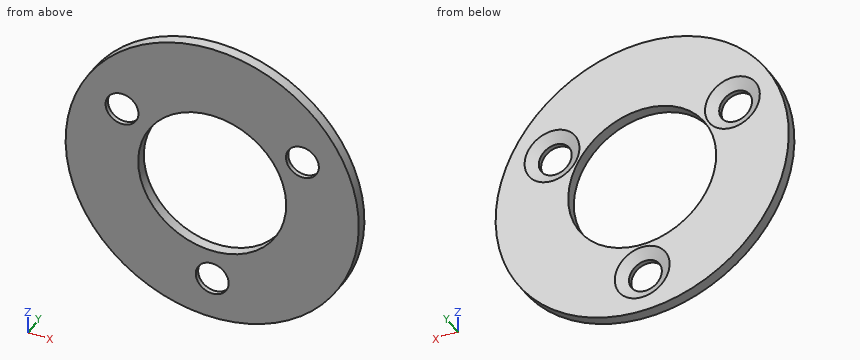
```python
from build123d import *

# Parameters (mm, degrees)
SKETCH_1_R          = 13.371753228
SKETCH_1_R_2        = 6.75
EXTRUDE_1_DEPTH     = 1
SKETCH_2_R          = 1.5
CUT_EXTRUDE_1_DEPTH = 2
CHAMFER_1_SIZE      = 1
CHAMFER_1_SIZE2     = 0.577350269


with BuildPart() as part:
    # 草图1 → 凸台-拉伸1 (new body)
    with BuildSketch(Plane(origin=(0, 0, 0), x_dir=(1, 0, 0), z_dir=(0, 1, 0))):
        with Locations(Location((0, 0, 0), (0, 0, 270))):
            Circle(SKETCH_1_R)
        with Locations(Location((0, 0, 0), (0, 0, 270))):
            Circle(SKETCH_1_R_2, mode=Mode.SUBTRACT)
    extrude(amount=EXTRUDE_1_DEPTH)

    # 草图2 → 切除-拉伸1 (cut)
    with BuildSketch(Plane(origin=(0, 1, 0), x_dir=(1, 0, 0), z_dir=(0, 1, 0))):
        with Locations(Location((0, 9.5, 0), (0, 0, 270))):
            Circle(SKETCH_2_R)
        with Locations(Location((8.227241336, -4.75, 0), (0, 0, 270))):
            Circle(SKETCH_2_R)
        with Locations(Location((-8.227241336, -4.75, 0), (0, 0, 270))):
            Circle(SKETCH_2_R)
    extrude(amount=-CUT_EXTRUDE_1_DEPTH, mode=Mode.SUBTRACT)

    # 倒角1
    chamfer_1_edges = [part.edges().sort_by_distance(p)[0] for p in [
        (0, 1, -11),
        (8.227241336, 1, 3.25),
        (-8.227241336, 1, 3.25),
    ]]
    chamfer_1_side = [part.faces().sort_by_distance(p)[0] for p in [
        (0, 1, -12.993542933),
    ]]
    chamfer(chamfer_1_edges, length=CHAMFER_1_SIZE, length2=CHAMFER_1_SIZE2, reference=chamfer_1_side[0])


solid = part.part
```
Here's how the part is built. I have some questions about the finished solid (model axes, mm). Give positions to 0.01 mm unless a question says otherwise; leave off trailing zeros. Loops run counter-clockwise (first coordinate to the right, second up) from the corner with the lowest first, then second, coordinate; pieces in that order, holes last. Notation, with made-up numbers: M -32,20 L 0,20 A11 cw 0,29 Z; hole C 26,56 d8. An arc over 180 degrees is marked long. Use one line per item in the form item = value. Start each with the question number.
Q1. If we section it at A-A (x = 0): Write out the boundary of the cut face in (y, z), then the cut area to 3 significant figures.
Q2. If we section it at D-D (z = 4.75): Write out the boundary of the cut face in (x, y), then the cut area to 3 significant figures.
Q3. If we section it at C-C (y = 0.6): Write out the boundary of the cut face in (x, z).
Q4. I need wall thicknesses on line 1 along X through (y, z) = (0.75, 0); line 2 along X through (y, z) = (0.8, 2.5); line 3 along Z through (x, y) = (9, 0.35). Which ranges of each line are inside material? Lowest first, please.
Q5. If we section it at B-B (z = 0): Write out the boundary of the cut face in (x, y), then the cut area to 3 significant figures.
Taken from the geometry:
q1.outline = M 0,-13.37 L 1,-13.37 L 1,-12 L 0.42,-11 L 0,-11 Z; M 0,-8 L 0.42,-8 L 1,-7 L 1,-6.75 L 0,-6.75 Z; M 0,6.75 L 1,6.75 L 1,13.37 L 0,13.37 Z
q1.area = 9.67 mm^2
q2.outline = M -12.5,0 L -9.73,0 L -9.73,0.42 L -10.73,1 L -12.5,1 Z; M -6.73,0 L -4.8,0 L -4.8,1 L -5.73,1 L -6.73,0.42 Z; M 4.8,0 L 6.73,0 L 6.73,0.42 L 5.73,1 L 4.8,1 Z; M 9.73,0 L 12.5,0 L 12.5,1 L 10.73,1 L 9.73,0.42 Z
q2.area = 8.25 mm^2
q3.outline = C 0,0 d26.74; hole C -8.23,4.75 d3.61; hole C 0,0 d13.5; hole C 0,-9.5 d3.61; hole C 8.23,4.75 d3.61
q4.line_1 = -13.37 to -6.75, 6.75 to 13.37
q4.line_2 = -13.14 to -6.27, 6.27 to 13.14
q4.line_3 = -9.89 to 3.46, 6.04 to 9.89
q5.outline = M -13.37,0 L -6.75,0 L -6.75,1 L -13.37,1 Z; M 6.75,0 L 13.37,0 L 13.37,1 L 6.75,1 Z
q5.area = 13.2 mm^2
